Input: part model. Units: mm. Frame: model coordinates. A direction names the side the tool comes from. Round coordinates to 2 decimals unless told otherwise and drop trailing zeros. Loops run counter-clockwise (first coordinate to the right, second up) from the corner with the lowest first, then second, coordinate; pieces in that order, holes last.
(1) First-contact query: pin 1 Ø3.5 at (x, y) = (24, 0) entering from -Z; pin 2 Ø0.7 at (y, z) = (-1.5, 1.5) entering from +X; pin 3 Ø3 at (x, y) = (7, 0.5) entering from +Z (3 decimals); pin 4 Ø2.5 at (x, z) = (15, 0) entering from +Y. Flat tips, straight axial feed; report the tip coordinate or a pass-through.
(2) Draft query along Y for faces 6 (the face through (-3.7, 0.1, 0.1)), 7 (the face through (3.413, -1.428, -0.055)), 8 (the face through (26.7, 4, 2)), 9 (the face through (26.59, -2.64, 0.05)). Return one class per face: released by +Y, released by -Y, zero draft, split by the parting line, or undercut.
(3) Cut plane D-D, the plane x = 8. Output: boundary loops of the cut face in (y, z) (3 decimals), and give its area (3 significant figures).
(4) Cut plane A-A, the plane x = 2.5. Output: boundary loops of the cut face in (y, z) (3 decimals), and give its area (3 significant figures).
(5) Cut plane B-B, the plane y = 6.25. Output: boundary loops of the cut face in (x, z) (3 decimals).
(6) Line query: line 1 (Y direction, x = 24, z = -3.45); line 2 (Y direction, x = 24, z = -1); line 3 (X direction, y = -1, z = 0.25). Output: solid intervals per line, ascending.
(7) Access query for faces 1 (the face through (-0.9, 2, 0)), 2 (the face through (20.3, 6, 0)), 3 (the face through (24, 4, 0.925)), 4 (the face through (12, -3.7, 0)), 5 (the face through (4.9, 0.1, -3.3)). Directions: +Z, -Z, +X, -X, +Y, -Y. A direction counts if a zero-diameter tool reaches every point of the face in a straight line with its end or side. Return the directions, or none.
(8) Cut plane C-C, the plane z = 0.5. Give the number of separate pieces and of enclosed holes in the cut face, and give its area (3 significant figures).
from build123d import *

# Parameters (mm, degrees)
SKETCH1_R            = 2.4
BEAM_DEPTH           = 3.925
AXLE_CUT_DEPTH       = 31.324670237
AXLE_CUT_DEPTH_BACK  = 31.324670237
SKETCH2_W            = 1.8
SKETCH2_H            = 1.8
SKETCH3_R            = 3.1
HOLE_SURROUND_DEPTH  = 1.25
CAVITY_CUT_DEPTH     = 3
FILLET2_R            = 0.5
FILLET2_OF_MIRROR2_R = 0.5
FILLET3_R            = 0.5


with BuildPart() as part:
    # Sketch1 → Beam (new, symmetric)
    with BuildSketch(Plane.XY):
        with BuildLine():
            Line((20.3, 3.7), (0, 3.7))
            ThreePointArc((0, 3.7), (-3.7, 0), (0, -3.7))
            Line((0, -3.7), (24, -3.7))
            ThreePointArc((24, -3.7), (26.61629509, -2.61629509), (27.7, 0))
            Line((27.7, 0), (27.7, 8))
            ThreePointArc((27.7, 8), (24, 11.7), (20.3, 8))
            Line((20.3, 8), (20.3, 3.7))
        make_face()
        with Locations((8, 0)):
            Circle(SKETCH1_R, mode=Mode.SUBTRACT)
        with Locations((16, 0)):
            Circle(SKETCH1_R, mode=Mode.SUBTRACT)
        with Locations((24, 0)):
            Circle(SKETCH1_R, mode=Mode.SUBTRACT)
        with Locations((24, 8)):
            Circle(SKETCH1_R, mode=Mode.SUBTRACT)
    extrude(amount=BEAM_DEPTH, both=True)

    # Sketch2 → Axle Cut (cut, two sides: drawn at the far end of the back side and taken through both)
    with BuildSketch(Plane.XY.offset(-AXLE_CUT_DEPTH_BACK)):
        Rectangle(SKETCH2_W, SKETCH2_H)
        with BuildLine():
            Line((-2.224859546, -0.9), (-0.9, -0.9))
            Line((-0.9, -0.9), (-0.9, 0.9))
            Line((-0.9, 0.9), (-2.224859546, 0.9))
            ThreePointArc((-2.224859546, 0.9), (-2.355808026, 0.45844143), (-2.4, 0))
            ThreePointArc((-2.4, 0), (-2.355808026, -0.45844143), (-2.224859546, -0.9))
        make_face()
        with BuildLine():
            Line((-0.9, 2.224859546), (-0.9, 0.9))
            Line((-0.9, 0.9), (0.9, 0.9))
            Line((0.9, 0.9), (0.9, 2.224859546))
            ThreePointArc((0.9, 2.224859546), (0.45844143, 2.355808026), (0, 2.4))
            ThreePointArc((0, 2.4), (-0.45844143, 2.355808026), (-0.9, 2.224859546))
        make_face()
        with BuildLine():
            Line((0.9, 0.9), (0.9, -0.9))
            Line((0.9, -0.9), (2.224859546, -0.9))
            ThreePointArc((2.224859546, -0.9), (2.355808026, -0.45844143), (2.4, 0))
            ThreePointArc((2.4, 0), (2.355808026, 0.45844143), (2.224859546, 0.9))
            Line((2.224859546, 0.9), (0.9, 0.9))
        make_face()
        with BuildLine():
            ThreePointArc((-0.9, -2.224859546), (-0.45844143, -2.355808026), (0, -2.4))
            ThreePointArc((0, -2.4), (0.45844143, -2.355808026), (0.9, -2.224859546))
            Line((0.9, -2.224859546), (0.9, -0.9))
            Line((0.9, -0.9), (-0.9, -0.9))
            Line((-0.9, -0.9), (-0.9, -2.224859546))
        make_face()
        with BuildLine():
            ThreePointArc((3.7, 0), (3.672112828, -0.453417441), (3.588871689, -0.9))
            ThreePointArc((3.588871689, -0.9), (3.188981578, -1.876271967), (2.529822128, -2.7))
            Line((2.529822128, -2.7), (5.470177872, -2.7))
            ThreePointArc((5.470177872, -2.7), (4.3, 0), (5.470177872, 2.7))
            Line((5.470177872, 2.7), (2.529822128, 2.7))
            ThreePointArc((2.529822128, 2.7), (3.188981578, 1.876271967), (3.588871689, 0.9))
            ThreePointArc((3.588871689, 0.9), (3.672112828, 0.453417441), (3.7, 0))
        make_face()
        with BuildLine():
            Line((2.4, 0), (2.4, -0.9))
            Line((2.4, -0.9), (3.588871689, -0.9))
            ThreePointArc((3.588871689, -0.9), (3.672112828, -0.453417441), (3.7, 0))
            ThreePointArc((3.7, 0), (3.672112828, 0.453417441), (3.588871689, 0.9))
            Line((3.588871689, 0.9), (2.4, 0.9))
            Line((2.4, 0.9), (2.4, 0))
        make_face()
        with BuildLine():
            ThreePointArc((2.224859546, 0.9), (2.355808026, 0.45844143), (2.4, 0))
            Line((2.4, 0), (2.4, 0.9))
            Line((2.4, 0.9), (2.224859546, 0.9))
        make_face()
        with BuildLine():
            ThreePointArc((2.4, 0), (2.355808026, -0.45844143), (2.224859546, -0.9))
            Line((2.224859546, -0.9), (2.4, -0.9))
            Line((2.4, -0.9), (2.4, 0))
        make_face()
    extrude(amount=AXLE_CUT_DEPTH + AXLE_CUT_DEPTH_BACK, mode=Mode.SUBTRACT)

    # Sketch3 → Hole Surround (cut)
    with BuildSketch(Plane.XY.offset(3.925)):
        with Locations((24, 8)):
            Circle(SKETCH3_R)
        with Locations((24, 0)):
            Circle(SKETCH3_R)
        with Locations((16, 0)):
            Circle(SKETCH3_R)
        with Locations((8, 0)):
            Circle(SKETCH3_R)
    hole_surround = extrude(amount=-HOLE_SURROUND_DEPTH, mode=Mode.SUBTRACT)

    # Sketch4 → Cavity Cut (cut)
    with BuildSketch(Plane.XY.offset(3.925)):
        with BuildLine():
            Line((21.6, 5.25), (21.6, 3.7))
            Line((21.6, 3.7), (21.6, 2.75))
            ThreePointArc((21.6, 2.75), (24.209981249, 3.643954977), (26.7, 2.456114818))
            Line((26.7, 2.456114818), (26.7, 5.543885182))
            ThreePointArc((26.7, 5.543885182), (24.209981249, 4.356045023), (21.6, 5.25))
        make_face()
        with BuildLine():
            ThreePointArc((21.543885182, -2.7), (20.356045023, -0.209981249), (21.25, 2.4))
            Line((21.25, 2.4), (20.3, 2.4))
            Line((20.3, 2.4), (18.75, 2.4))
            ThreePointArc((18.75, 2.4), (19.417601498, 1.281600562), (19.65, 0))
            ThreePointArc((19.65, 0), (19.338212028, -1.476089583), (18.456114818, -2.7))
            Line((18.456114818, -2.7), (21.543885182, -2.7))
        make_face()
        with BuildLine():
            ThreePointArc((13.543885182, -2.7), (12.356045023, -0.209981249), (13.25, 2.4))
            Line((13.25, 2.4), (10.75, 2.4))
            ThreePointArc((10.75, 2.4), (11.417601498, 1.281600562), (11.65, 0))
            ThreePointArc((11.65, 0), (11.338212028, -1.476089583), (10.456114818, -2.7))
            Line((10.456114818, -2.7), (13.543885182, -2.7))
        make_face()
        with BuildLine():
            Line((10.75, 2.4), (13.25, 2.4))
            ThreePointArc((13.25, 2.4), (13.392624332, 2.554230241), (13.543885182, 2.7))
            Line((13.543885182, 2.7), (10.456114818, 2.7))
            ThreePointArc((10.456114818, 2.7), (10.607375668, 2.554230241), (10.75, 2.4))
        make_face()
    cavity_cut = extrude(amount=-CAVITY_CUT_DEPTH, mode=Mode.SUBTRACT)

    # Fillet2
    fillet2_edges = [part.edges().sort_by_distance(p)[0] for p in [
        (26.7, 2.456114818, 2.425),
        (21.6, 2.75, 2.425),
        (21.6, 5.25, 2.425),
        (26.7, 5.543885182, 2.425),
        (18.456114818, -2.7, 2.425),
        (18.75, 2.4, 2.425),
        (21.25, 2.4, 2.425),
        (21.543885182, -2.7, 2.425),
        (10.456114818, -2.7, 2.425),
        (10.456114818, 2.7, 2.425),
        (13.543885182, 2.7, 2.425),
        (13.543885182, -2.7, 2.425),
    ]]
    fillet(fillet2_edges, radius=FILLET2_R)

    # Mirror2: Hole Surround, Cavity Cut across plane
    add(hole_surround.mirror(Plane.XY), mode=Mode.SUBTRACT)
    add(cavity_cut.mirror(Plane.XY), mode=Mode.SUBTRACT)

    # Fillet2 of Mirror2
    fillet2_of_mirror2_edges = [part.edges().sort_by_distance(p)[0] for p in [
        (26.7, 2.456114818, -2.425),
        (21.6, 2.75, -2.425),
        (21.6, 5.25, -2.425),
        (26.7, 5.543885182, -2.425),
        (18.456114818, -2.7, -2.425),
        (18.75, 2.4, -2.425),
        (21.25, 2.4, -2.425),
        (21.543885182, -2.7, -2.425),
        (10.456114818, -2.7, -2.425),
        (10.456114818, 2.7, -2.425),
        (13.543885182, 2.7, -2.425),
        (13.543885182, -2.7, -2.425),
    ]]
    fillet(fillet2_of_mirror2_edges, radius=FILLET2_OF_MIRROR2_R)

    # Fillet3
    fillet3_edges = [part.edges().sort_by_distance(p)[0] for p in [
        (2.529822128, 2.7, 0),
        (5.470177872, 2.7, 0),
        (5.470177872, -2.7, 0),
        (2.529822128, -2.7, 0),
    ]]
    fillet(fillet3_edges, radius=FILLET3_R)


solid = part.part
Reported:
1. pin 1: passes through
1. pin 2: stops at x = 27.52
1. pin 3: stops at z = 2.675
1. pin 4: stops at y = 3.7
2. face 6: split by the parting line
2. face 7: undercut
2. face 8: undercut
2. face 9: released by -Y
3. outline: (-3.7, -3.925) - (-3.1, -3.925) - (-3.1, -2.675) - (-2.4, -2.675) - (-2.4, 2.675) - (-3.1, 2.675) - (-3.1, 3.925) - (-3.7, 3.925) - close; (2.4, -2.675) - (3.1, -2.675) - (3.1, -3.925) - (3.7, -3.925) - (3.7, 3.925) - (3.1, 3.925) - (3.1, 2.675) - (2.4, 2.675) - close
3. area: 16.9 mm2
4. outline: (-3.7, -3.925) - (-0.9, -3.925) - (-0.9, 3.925) - (-3.7, 3.925) - close; (0.9, -3.925) - (3.7, -3.925) - (3.7, 3.925) - (0.9, 3.925) - close
4. area: 44.0 mm2
5. outline: (20.3, -3.925) - (21.441, -3.925) - (21.441, -2.675) - (22.358, -2.675) - (22.358, 2.675) - (21.441, 2.675) - (21.441, 3.925) - (20.3, 3.925) - close; (25.642, -2.675) - (26.559, -2.675) - (26.559, -3.925) - (27.7, -3.925) - (27.7, 3.925) - (26.559, 3.925) - (26.559, 2.675) - (25.642, 2.675) - close
6. line 1: y = -3.7 to -3.1, 3.1 to 3.65, 4.35 to 4.9, 11.1 to 11.7
6. line 2: y = -3.7 to -2.4, 2.4 to 3.65, 4.35 to 5.6, 10.4 to 11.7
6. line 3: x = -3.56 to -0.9, 0.9 to 3.56, 4.44 to 5.82, 10.18 to 13.82, 18.18 to 21.82, 26.18 to 27.56
7. face 1: +Z, -Z
7. face 2: +Z, -Z, -X, +Y
7. face 3: +Z
7. face 4: +Z, -Z, +X, -X, -Y
7. face 5: -Z
8. separate pieces: 1
8. enclosed holes: 5
8. area: 182 mm2
